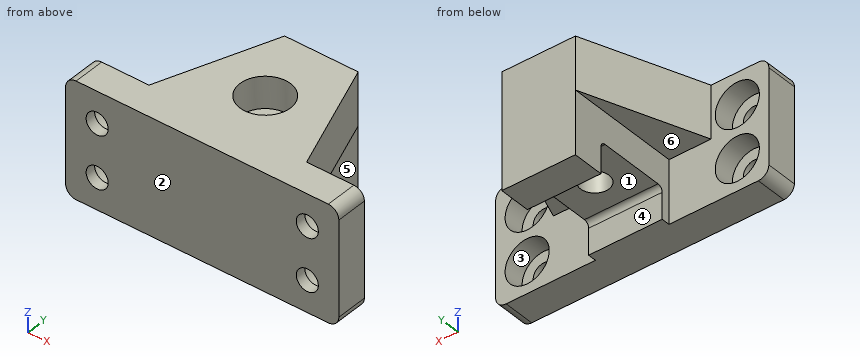
from build123d import *

# Parameters (mm, degrees)
SKETCH1_W           = 26
SKETCH1_H           = 11
SKETCH1_R           = 1.05
BOSS_EXTRUDE1_DEPTH = 3
SKETCH10_R          = 2.1
CUT_EXTRUDE6_DEPTH  = 2
SKETCH3_W           = 7
SKETCH3_H           = 14
BOSS_EXTRUDE2_DEPTH = 11
SKETCH6_W           = 3
SKETCH6_H           = 7.2
CUT_EXTRUDE3_DEPTH  = 23.327113562
SKETCH7_R           = 1.35
CUT_EXTRUDE4_DEPTH  = 21.712315177
SKETCH8_R           = 2.4
CUT_EXTRUDE5_DEPTH  = 3
FILLET1_R           = 0.5
FILLET2_R           = 1
BOSS_EXTRUDE3_DEPTH = 5


with BuildPart() as part:
    # Sketch1 → Boss-Extrude1 (new body)
    with BuildSketch(Plane(origin=(0, 0, 0), x_dir=(1, 0, 0), z_dir=(0, 1, 0))):
        Rectangle(SKETCH1_W, SKETCH1_H)
        with Locations(Location((-10, 2.5, 0), (0, 0, 270))):
            Circle(SKETCH1_R, mode=Mode.SUBTRACT)
        with Locations(Location((-10, -2.5, 0), (0, 0, 270))):
            Circle(SKETCH1_R, mode=Mode.SUBTRACT)
        with Locations(Location((10, 2.5, 0), (0, 0, 270))):
            Circle(SKETCH1_R, mode=Mode.SUBTRACT)
        with Locations(Location((10, -2.5, 0), (0, 0, 270))):
            Circle(SKETCH1_R, mode=Mode.SUBTRACT)
    extrude(amount=BOSS_EXTRUDE1_DEPTH)

    # Sketch10 → Cut-Extrude6 (cut)
    with BuildSketch(Plane(origin=(0, 3, 0), x_dir=(1, 0, 0), z_dir=(0, 1, 0))):
        with Locations(Location((-10, 2.5, 0), (0, 0, 270))):
            Circle(SKETCH10_R)
        with Locations(Location((-10, -2.5, 0), (0, 0, 270))):
            Circle(SKETCH10_R)
        with Locations(Location((10, 2.5, 0), (0, 0, 270))):
            Circle(SKETCH10_R)
        with Locations(Location((10, -2.5, 0), (0, 0, 270))):
            Circle(SKETCH10_R)
    extrude(amount=-CUT_EXTRUDE6_DEPTH, mode=Mode.SUBTRACT)

    # Sketch3 → Boss-Extrude2 (add)
    with BuildSketch(Plane(origin=(0, 0, -5.5), x_dir=(-1, 0, 0), z_dir=(0, 0, -1))):
        with Locations((0, 7)):
            Rectangle(SKETCH3_W, SKETCH3_H)
    extrude(amount=-BOSS_EXTRUDE2_DEPTH)

    # Sketch6 → Cut-Extrude3 (cut, through all)
    with BuildSketch(Plane(origin=(3.5, 0, 0), x_dir=(0, 0, -1), z_dir=(1, 0, 0))):
        with Locations((4, 7.4)):
            Rectangle(SKETCH6_W, SKETCH6_H)
    extrude(amount=-CUT_EXTRUDE3_DEPTH, mode=Mode.SUBTRACT)

    # Sketch7 → Cut-Extrude4 (cut, through all)
    with BuildSketch(Plane(origin=(0, 0, -2.5), x_dir=(-1, 0, 0), z_dir=(0, 0, -1))):
        with Locations(Location((0, 7.4, 0), (0, 0, 90))):
            Circle(SKETCH7_R)
    extrude(amount=-CUT_EXTRUDE4_DEPTH, mode=Mode.SUBTRACT)

    # Sketch8 → Cut-Extrude5 (cut)
    with BuildSketch(Plane.XY.offset(5.5)):
        with Locations((0, 7.4)):
            Circle(SKETCH8_R)
    extrude(amount=-CUT_EXTRUDE5_DEPTH, mode=Mode.SUBTRACT)

    # Fillet1
    fillet1_edges = [part.edges().sort_by_distance(p)[0] for p in [
        (0, 3.8, -2.5),
        (0, 11, -2.5),
    ]]
    fillet(fillet1_edges, radius=FILLET1_R)

    # Fillet2
    fillet2_edges = [part.edges().sort_by_distance(p)[0] for p in [
        (13, 1.5, 5.5),
        (-13, 1.5, 5.5),
        (-13, 1.5, -5.5),
        (13, 1.5, -5.5),
    ]]
    fillet(fillet2_edges, radius=FILLET2_R)

    # Sketch9 → Boss-Extrude3 (add)
    with BuildSketch(Plane.XY.offset(5.5)):
        Polygon((3.5, 3), (3.5, 14), (7.5, 3), align=None)
        Polygon((-7.5, 3), (-3.5, 3), (-3.5, 14), align=None)
    extrude(amount=-BOSS_EXTRUDE3_DEPTH)


solid = part.part
Build history of the part. All positions in model axes, mm. Face numbers are marked on the shaded views. A direction names the side the tool comes from. Round coordinates to 2 decimals unless told otherwise and drop trailing zeros. Loops run counter-clockwise (first coordinate to the right, second up) from the corner with the lowest first, then second, coordinate; pieces in that order, holes last. Notation, with made-up numbers: (85, -23.75) -> (122, -23.75) arc R5 ccw to (122, -19.75) -> close; hole circle Ø10 at (-12, 55.25). An arc over 180 degrees is marked (long way). Answer in a Markdown table with one row per item.
Item 1: Saw through at C-C (y = 1.75). Write the cut outline in (x, z), and give its area (3 significant figures).
Answers below:
| item | result |
|---|---|
| outline | (-13, -4.5) arc R1 ccw to (-12, -5.5) -> (12, -5.5) arc R1 ccw to (13, -4.5) -> (13, 4.5) arc R1 ccw to (12, 5.5) -> (-12, 5.5) arc R1 ccw to (-13, 4.5) -> close; hole circle Ø4.2 at (-10, -2.5); hole circle Ø4.2 at (-10, 2.5); hole circle Ø4.2 at (10, -2.5); hole circle Ø4.2 at (10, 2.5) |
| area | 230 mm² |
Item 2: Pin check, flat tips, straight feed: pin 1 (4 mm diameter, centred on x = -10, z = -2.5, fed in from -Y); pin 2 (5 mm diameter, centred on x = 0, y = 8, fed in from -Z); pin 3 (1.9 mm diameter, centred on x = 10, z = 2.5, fed in from +Y); pin 4 (3.5 mm diameter, centred on x = -10, z = -2.5, fed in from +Y). Stop position of each tip, or through.
Answers below:
| item | result |
|---|---|
| pin 1 | stops at y = 0 |
| pin 2 | stops at z = -2.5 |
| pin 3 | passes through |
| pin 4 | stops at y = 1 |
Item 3: Mould opens along Z. For the marked faces 1, 2 and 3 say: +Z half, -Z half, draft (parallel to the pull), parting line (faces both ways), or undercut.
Answers below:
| item | result |
|---|---|
| face 1 | -Z half |
| face 2 | draft |
| face 3 | undercut |
Item 4: Saw through at D-D (x = 1). Write the cut outline in (y, z).
Answers below:
| item | result |
|---|---|
| outline | (0, -5.5) -> (3.8, -5.5) -> (3.8, -3) arc R0.5 cw to (4.3, -2.5) -> (6.49, -2.5) -> (6.49, 2.5) -> (5.22, 2.5) -> (5.22, 5.5) -> (0, 5.5) -> close; (8.31, -2.5) -> (10.5, -2.5) arc R0.5 cw to (11, -3) -> (11, -5.5) -> (14, -5.5) -> (14, 5.5) -> (9.58, 5.5) -> (9.58, 2.5) -> (8.31, 2.5) -> close |
Item 5: Which spindle directions (+Z, -Z, +X, -X, +Y, -Y) get a long thin tool onto all of the face, cutting with end or side? Do the marked faces 4, 5 and 6. Say none if no direction does.
Answers below:
| item | result |
|---|---|
| face 4 | -Z, +X, -X |
| face 5 | -Z, +X, +Y |
| face 6 | -Z, -X, +Y |
Item 6: Saw through at A-A (y = 7.4). Write the cut outline in (x, z).
Answers below:
| item | result |
|---|---|
| outline | (-5.9, 0.5) -> (-3.5, 0.5) -> (-3.5, -2.5) -> (-1.35, -2.5) -> (-1.35, 2.5) -> (-2.4, 2.5) -> (-2.4, 5.5) -> (-5.9, 5.5) -> close; (1.35, -2.5) -> (3.5, -2.5) -> (3.5, 0.5) -> (5.9, 0.5) -> (5.9, 5.5) -> (2.4, 5.5) -> (2.4, 2.5) -> (1.35, 2.5) -> close |
Item 7: Saw through at B-B (x = -10). Write the cut outline in (y, z).
Answers below:
| item | result |
|---|---|
| outline | (0, -5.5) -> (3, -5.5) -> (3, -4.6) -> (1, -4.6) -> (1, -3.55) -> (0, -3.55) -> close; (0, -1.45) -> (1, -1.45) -> (1, -0.4) -> (3, -0.4) -> (3, 0.4) -> (1, 0.4) -> (1, 1.45) -> (0, 1.45) -> close; (0, 3.55) -> (1, 3.55) -> (1, 4.6) -> (3, 4.6) -> (3, 5.5) -> (0, 5.5) -> close |
Item 8: Drill centre lines: L1, parallel to X at y = 0.6, z = 2.5; L2, parallel to Z at x = 10, y = 0.4; L3, parallel to X at y = 1.5, z = 2.5. Where is each one in solid material? Low to high. Write a range as [from, to].
Answers below:
| item | result |
|---|---|
| L1 | x = [-13, -11.05], [-8.95, 8.95], [11.05, 13] |
| L2 | z = [-5.5, -3.55], [-1.45, 1.45], [3.55, 5.5] |
| L3 | x = [-13, -12.1], [-7.9, 7.9], [12.1, 13] |
